Part model, mm, in its own coordinate system. Face numbers are marked on the shaded views. Coordinates: 2 decimals unless noted, no trailing zeros. Loops run counter-clockwise (first coordinate to the right, second up) from the corner with the lowest first, then second, coordinate; pieces in that order, holes last. Notation, with made-up numbers: (15, 83) -> (24, 83) arc R27 ccw to (24, 113) -> close; hole circle Ø10 at (83, -10). An arc over 180 degrees is marked (long way). Use one line per item in the form item = value. Start each with the question number.
(1) Mould opens along Y. For the marked faces 1, 2 and 3 say: +Y half, -Y half, draft (parallel to the pull), parting line (faces both ways), or undercut.
(2) Band-saw the part on C-C on y = -2.5. Count the separate pieces of the cut face and the enclosed holes in it, then the cut area to 3 significant figures.
(3) Drill centre lines: L1, parallel to Y at x = 0, z = -69.5; L2, parallel to Y at x = 18, z = -152. Where is each one in solid material? Low to high. Write a range as [from, to].
(4) Pin check, flat tip, straight feed: P1, Ø9, axis at y = -2, z = -102, coming from the -X side. Stop position of the tip, or through.
(5) Band-saw the part on A-A on x = -11. Give the cut face in (y, z), then the cut area to 3 significant figures.
```python
from build123d import *

# Parameters (mm, degrees)
EXTRUDE_THIN1_DEPTH = 304.8
FILLET2_R           = 0.762
FILLET3_R           = 1.524
SKETCH4_R           = 5.08
CUT_EXTRUDE1_DEPTH  = 309.273534432
CHAMFER1_SIZE       = 0.635


with BuildPart() as part:
    # Sketch1 → Extrude-Thin1 (new body)
    with BuildSketch(Plane.XY):
        with BuildLine():
            Line((-13.5255, 9.525), (-18.2499, 9.525))
            ThreePointArc((-18.2499, 9.525), (-19.938188151, 10.224311849), (-20.6375, 11.9126))
            Line((-20.6375, 11.9126), (-20.6375, 18.2499))
            ThreePointArc((-20.6375, 18.2499), (-19.938188151, 19.938188151), (-18.2499, 20.6375))
            Line((-18.2499, 20.6375), (18.2499, 20.6375))
            ThreePointArc((18.2499, 20.6375), (19.938188151, 19.938188151), (20.6375, 18.2499))
            Line((20.6375, 18.2499), (20.6375, -18.2499))
            ThreePointArc((20.6375, -18.2499), (19.938188151, -19.938188151), (18.2499, -20.6375))
            Line((18.2499, -20.6375), (-18.2499, -20.6375))
            ThreePointArc((-18.2499, -20.6375), (-19.938188151, -19.938188151), (-20.6375, -18.2499))
            Line((-20.6375, -18.2499), (-20.6375, -11.9126))
            ThreePointArc((-20.6375, -11.9126), (-19.938188151, -10.224311849), (-18.2499, -9.525))
            Line((-18.2499, -9.525), (-13.5255, -9.525))
            Line((-13.5255, -9.525), (-13.5255, -13.589))
            Line((-13.5255, -13.589), (-16.5735, -13.589))
            Line((-16.5735, -13.589), (-16.5735, -16.5735))
            Line((-16.5735, -16.5735), (16.5735, -16.5735))
            Line((16.5735, -16.5735), (16.5735, 16.5735))
            Line((16.5735, 16.5735), (-16.5735, 16.5735))
            Line((-16.5735, 16.5735), (-16.5735, 13.589))
            Line((-16.5735, 13.589), (-13.5255, 13.589))
            Line((-13.5255, 13.589), (-13.5255, 9.525))
        make_face()
    extrude(amount=-EXTRUDE_THIN1_DEPTH)

    # Fillet2
    fillet2_edges = [part.edges().sort_by_distance(p)[0] for p in [
        (-16.5735, -13.589, -152.4),
        (-16.5735, -16.5735, -152.4),
        (-16.5735, 16.5735, -152.4),
        (-16.5735, 13.589, -152.4),
        (-13.5255, 13.589, -152.4),
        (-13.5255, 9.525, -152.4),
        (-13.5255, -9.525, -152.4),
        (-13.5255, -13.589, -152.4),
    ]]
    fillet(fillet2_edges, radius=FILLET2_R)

    # Fillet3
    fillet3_edges = [part.edges().sort_by_distance(p)[0] for p in [
        (16.5735, -16.5735, -152.4),
        (16.5735, 16.5735, -152.4),
    ]]
    fillet(fillet3_edges, radius=FILLET3_R)

    # Sketch4 → Cut-Extrude1 (cut, through all)
    with BuildSketch(Plane(origin=(20.6375, 0, 0), x_dir=(0, 0, -1), z_dir=(1, 0, 0))):
        with Locations((152.4, 0)):
            Circle(SKETCH4_R)
        with Locations((184.15, 0)):
            Circle(SKETCH4_R)
        with Locations((120.65, 0)):
            Circle(SKETCH4_R)
    extrude(amount=-CUT_EXTRUDE1_DEPTH, mode=Mode.SUBTRACT)

    # Chamfer1
    chamfer1_edges = [part.edges().sort_by_distance(p)[0] for p in [
        (20.6375, 0, -115.57),
        (16.5735, 0, -179.07),
        (20.6375, 0, -179.07),
    ]]
    chamfer(chamfer1_edges, length=CHAMFER1_SIZE)


solid = part.part
```
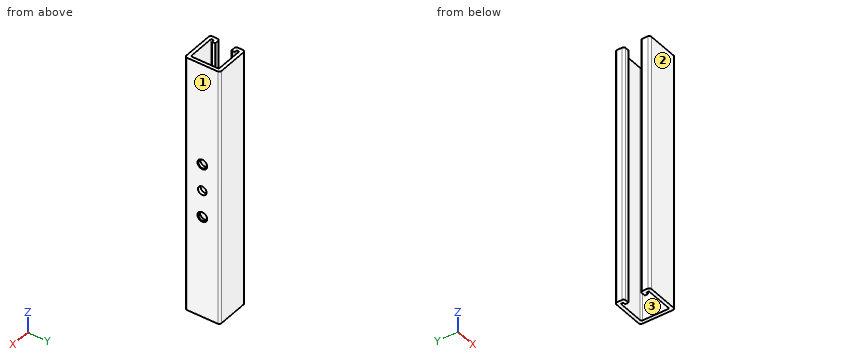
A:
q1.face_1 = draft
q1.face_2 = -Y half
q1.face_3 = undercut
q2.separate_pieces = 4
q2.enclosed_holes = 0
q2.area = 1,130 mm²
q3.L1 = [-20.64, -16.57], [16.57, 20.64]
q3.L2 = [-20.64, -5.06], [5.06, 20.64]
q4.P1 = 16.57
q5.outline = (-20.64, -304.8) -> (-16.57, -304.8) -> (-16.57, 0) -> (-20.64, 0) -> close; (16.57, -304.8) -> (20.64, -304.8) -> (20.64, 0) -> (16.57, 0) -> close
q5.area = 2,480 mm²
